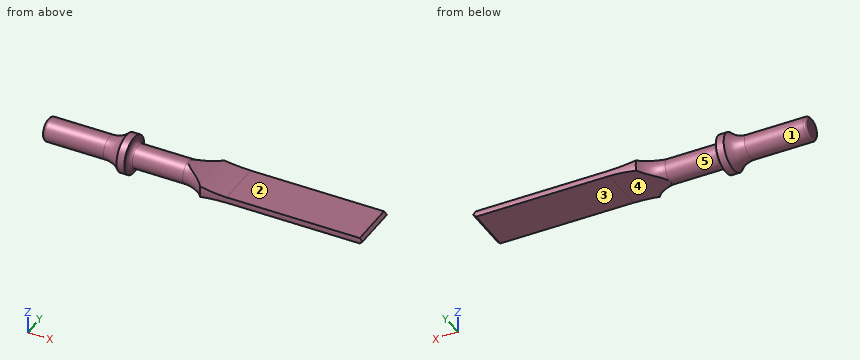
```python
from build123d import *

# Parameters (mm, degrees)
F3_DEPTH = 25
F4_DEPTH = 25


with BuildPart() as f1:
    # F0 (on Front) → F1 (revolve)
    with BuildSketch(Plane.XZ):
        with BuildLine():
            Line((0, 1.9), (0, 0))
            Line((0, 0), (70.28609, 0))
            Line((70.28609, 0), (70.28609, 5))
            Line((70.28609, 5), (35.28609, 5))
            ThreePointArc((35.28609, 5), (33.081175, 3.15983), (30.28609, 2.5))
            Line((30.28609, 2.5), (19.44, 2.5))
            ThreePointArc((19.44, 2.5), (18.803604, 2.763604), (18.54, 3.4))
            Line((18.54, 3.4), (18.54, 4.06))
            Line((18.54, 4.06), (16.87, 4.06))
            ThreePointArc((16.87, 4.06), (15.216288, 2.906526), (13.241447, 2.5))
            Line((13.241447, 2.5), (0.6, 2.5))
            ThreePointArc((0.6, 2.5), (0.175736, 2.324264), (0, 1.9))
        make_face()
    revolve(axis=Axis((35.143045, 0, 0), (1, 0, 0)))

    # F2 (on Front) → F3 (cut)
    with BuildSketch(Plane.XZ):
        with BuildLine():
            ThreePointArc((30.28609, 2.5), (35.579623, 1.146564), (41.018965, 0.63))
            Line((41.018965, 0.63), (69.65609, 0.63))
            Line((69.65609, 0.63), (70.28609, 0))
            Line((70.28609, 0), (73.746532, 14.08634))
            Line((73.746532, 14.08634), (30.28609, 14.08634))
            Line((30.28609, 14.08634), (30.28609, 2.5))
        make_face()
        with BuildLine():
            Line((73.746532, -14.08634), (70.28609, 0))
            Line((70.28609, 0), (69.65609, -0.63))
            Line((69.65609, -0.63), (41.018965, -0.63))
            ThreePointArc((41.018965, -0.63), (35.579623, -1.146564), (30.28609, -2.5))
            Line((30.28609, -2.5), (30.28609, -14.08634))
            Line((30.28609, -14.08634), (73.746532, -14.08634))
        make_face()
    extrude(amount=-F3_DEPTH, mode=Mode.SUBTRACT)

    # F2 (on Front) → F4 (cut)
    with BuildSketch(Plane.XZ):
        with BuildLine():
            ThreePointArc((30.28609, 2.5), (35.579623, 1.146564), (41.018965, 0.63))
            Line((41.018965, 0.63), (69.65609, 0.63))
            Line((69.65609, 0.63), (70.28609, 0))
            Line((70.28609, 0), (73.746532, 14.08634))
            Line((73.746532, 14.08634), (30.28609, 14.08634))
            Line((30.28609, 14.08634), (30.28609, 2.5))
        make_face()
        with BuildLine():
            Line((73.746532, -14.08634), (70.28609, 0))
            Line((70.28609, 0), (69.65609, -0.63))
            Line((69.65609, -0.63), (41.018965, -0.63))
            ThreePointArc((41.018965, -0.63), (35.579623, -1.146564), (30.28609, -2.5))
            Line((30.28609, -2.5), (30.28609, -14.08634))
            Line((30.28609, -14.08634), (73.746532, -14.08634))
        make_face()
    extrude(amount=F4_DEPTH, mode=Mode.SUBTRACT)


solid = f1.part
```
Check sheet for the modelled part. Datum: model origin and axes. Units: mm. Face numbers are marked on the shaded views. A direction names the side the tool comes from. Round coordinates to 2 decimals unless told otherwise and drop trailing zeros. Write each loop counter-clockwise with the first axis right and the second up, starting at its lowest first coordinate (ties: lowest second). Pieces come first, ordered by that corner, then holes. Notation, with made-up numbers: M 35.25,44 L 76.25,44 A31 cw 76.25,76 Z; hole C -6,6.5 d5. An arc over 180 degrees is marked long. Write item = value, one per line. Start each with the question number.
1. Tool access check on the marked faces 1 and 2. Record the directions out of +Z, -Z, +X, -X, +Y, -Y that give a thin tool (end or side, any length) a straight path to the whole face; none if there is none.
2. Gauge pin test, flat ends, axial feed: pin 1 (1 mm diameter, centred on x = 54.5, y = -2.5, fed in from +Z); pin 2 (2.5 mm diameter, centred on y = -2, z = -1, fed in from +X); pin 3 (5 mm diameter, centred on x = 15, y = 0, fed in from -Z); pin 4 (3 mm diameter, centred on x = 29, y = -2.5, fed in from +Z). Record the tip position at first contact, or that the pin passes through.
3. Scan lines: line 1 (Z direction, x = 53.5, y = 0.25); line 2 (X direction, y = 2, z = 2.5); line 3 (Z direction, x = 25, y = -2.25). Record each from-to range of solid material in increasing order. Write a range as [from, to].
4. Section check A-A, the plane x = 12.5. Record the cut outline in (y, z).
5. Release check for a two-part mould opening along X. For the marked faces 3, 4 and 5 record: pulls with the +X half, pulls with the -X half, needs draft (parallel to the pull), parting line crosses it, or undercut.
6. Section check C-C, the plane x = 40. Record the cut outline in (y, z), then the cut area to 3 significant figures.
7. Section check B-B, the plane x = 51.5. Record the cut outline in (y, z), then the cut area to 3 significant figures.
Results found:
q1.face_1 = -X
q1.face_2 = +Z, +X, +Y, -Y
q2.pin_1 = 0.63
q2.pin_2 = 70.29
q2.pin_3 = -4.06
q2.pin_4 = 2.29
q3.line_1 = [-0.63, 0.63]
q3.line_2 = [15.8, 18.56]
q3.line_3 = [-1.09, 1.09]
q4.outline = C 0,0 d5
q5.face_3 = needs draft
q5.face_4 = pulls with the +X half
q5.face_5 = undercut
q6.outline = M -4.96,-0.66 L 4.96,-0.66 A5 ccw 4.96,0.66 L -4.96,0.66 A5 ccw Z
q6.area = 13.2 mm^2
q7.outline = M -4.96,-0.63 L 4.96,-0.63 A5 ccw 4.96,0.63 L -4.96,0.63 A5 ccw Z
q7.area = 12.6 mm^2
